from build123d import *

# Parameters (mm, degrees)
BOSS_EXTRUDE1_DEPTH = 3.175
SKETCH4_W           = 17.018
SKETCH4_H           = 3.175
SKETCH4_H_2         = 3.144138513
SKETCH4_W_2         = 3.937
SKETCH4_W_3         = 12.7
CUT_EXTRUDE1_DEPTH  = 3.175
SKETCH5_W           = 7.516860114
SKETCH5_H           = 3.175
CUT_EXTRUDE2_DEPTH  = 3.175
SKETCH6_R           = 1.0287
CUT_EXTRUDE3_DEPTH  = 3.175
CUT_EXTRUDE4_DEPTH  = 4.064


with BuildPart() as part:
    # Sketch2 → Boss-Extrude1 (new body)
    with BuildSketch(Plane.XY):
        Polygon((-71.3232, 6.731), (11.7348, 6.731), (11.7348, 25.781), align=None)
        Polygon((11.7348, 25.781), (11.7348, 6.731), (71.3232, 6.731), align=None)
        Polygon((11.7348, 6.731), (11.7348, -6.731), (71.3232, -6.731), (71.3232, -4.699), (67.2592, -4.699), (67.2592, -1.143), (71.3232, -1.143), (71.3232, 0.381), (67.2592, 0.381), (67.2592, 3.937), (71.3232, 3.937), (71.3232, 4.572927428), (71.3232, 6.731), align=None)
        Polygon((-71.3232, -6.731), (11.7348, -6.731), (11.7348, 6.731), (-71.3232, 6.731), (-71.3232, 3.937), (-67.2592, 3.937), (-67.2592, 0.381), (-71.3232, 0.381), (-71.3232, -1.143), (-67.2592, -1.143), (-67.2592, -4.699), (-71.3232, -4.699), align=None)
    extrude(amount=BOSS_EXTRUDE1_DEPTH)

    # Sketch4 → Cut-Extrude1 (cut)
    with BuildSketch(Plane.XY.offset(3.175)):
        with Locations((-45.7962, -5.1435)):
            Rectangle(SKETCH4_W, SKETCH4_H)
        with Locations((-11.7602, -5.1435)):
            Rectangle(SKETCH4_W, SKETCH4_H)
        with Locations((22.2758, -5.158930744)):
            Rectangle(SKETCH4_W, SKETCH4_H_2)
        with Locations((75.1713, -5.1435)):
            Rectangle(SKETCH4_W_2, SKETCH4_H)
        with Locations((54.1528, -5.158930744)):
            Rectangle(SKETCH4_W_3, SKETCH4_H_2)
    extrude(amount=-CUT_EXTRUDE1_DEPTH, mode=Mode.SUBTRACT)

    # Sketch5 → Cut-Extrude2 (cut)
    with BuildSketch(Plane.XY.offset(3.175)):
        with Locations((68.198230057, -5.1435)):
            Rectangle(SKETCH5_W, SKETCH5_H)
    extrude(amount=-CUT_EXTRUDE2_DEPTH, mode=Mode.SUBTRACT)

    # Sketch6 → Cut-Extrude3 (cut)
    with BuildSketch(Plane.XY.offset(3.175)):
        with Locations((-61.9252, -1.8542)):
            Circle(SKETCH6_R)
        with Locations((-58.378607788, -1.8542)):
            Circle(SKETCH6_R)
        with Locations(Location((61.9252, -1.8542, 0), (0, 0, 180))):
            Circle(SKETCH6_R)
        with Locations(Location((58.378607788, -1.8542, 0), (0, 0, 180))):
            Circle(SKETCH6_R)
    extrude(amount=-CUT_EXTRUDE3_DEPTH, mode=Mode.SUBTRACT)

    # Sketch7 → Cut-Extrude4 (cut)
    with BuildSketch(Plane.XY.offset(3.175)):
        Polygon((-63.896048939, 8.434475014), (-57.706756389, 9.854037525), (-56.996975133, 6.75939125), (-63.186267684, 5.339828739), align=None)
        Polygon((-47.803888308, 12.125337544), (-32.949586187, 15.532287572), (-32.239804931, 12.437641297), (-47.094107052, 9.030691269), align=None)
        Polygon((-23.046718106, 17.80358759), (-16.857425556, 19.223150102), (-16.1476443, 16.128503827), (-22.33693685, 14.708941315), align=None)
        Polygon((-6.954557475, 21.49445012), (-0.765264924, 22.914012632), (-0.055483668, 19.819366357), (-6.244776219, 18.399803845), align=None)
        Polygon((24.145430883, 21.813407007), (30.193862821, 19.879765083), (29.227041859, 16.855549114), (23.178609921, 18.789191038), align=None)
        Polygon((36.242294759, 17.946123159), (42.290726697, 16.012481235), (41.323905735, 12.988265266), (35.275473797, 14.92190719), align=None)
        Polygon((47.129472248, 14.465567696), (53.177904186, 12.531925772), (52.211083224, 9.507709803), (46.162651286, 11.441351727), align=None)
        Polygon((58.016649736, 10.985012233), (64.065081674, 9.051370309), (63.098260712, 6.02715434), (57.049828774, 7.960796264), align=None)
    extrude(amount=-CUT_EXTRUDE4_DEPTH, mode=Mode.SUBTRACT)


solid = part.part
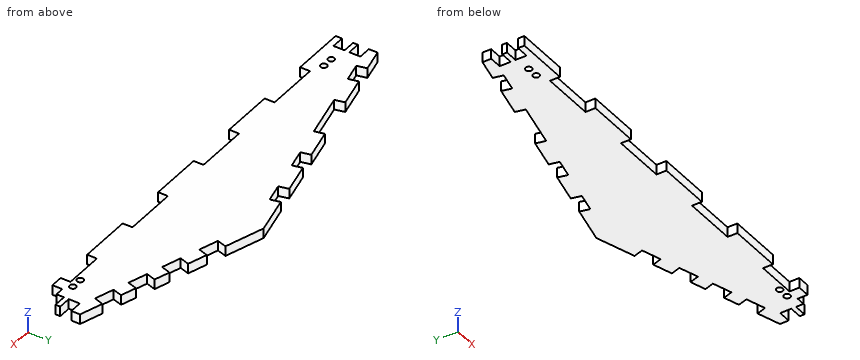
Work out the finished part from the listing and answer in its coordinate system (mm). Give positions to 0.01 mm unless a question says otherwise; leave off trailing zeros. Order: outer loops, then holes, each group sorted by start corner. A loop starts at its lowest first (then second) coordinate and runs counter-clockwise, first axis right, second up. Notation, with made-up numbers: (44, 75) -> (89, 75) arc R11 cw to (89, 80) -> close; hole circle Ø8 at (34.25, 69.5). An arc over 180 degrees is marked (long way). Answer as a JSON object with one key per item and string values. Group by question number.
1. Section A-A on z = 0.65 is taken. Count the separate pieces of the cut face and the enclosed holes in it, plus the area to 3 significant figures.
2. Section B-B on x = 32 is taken. Determine the outline of the cut face in (y, z) (3 decimals).
3. Flat-ended cylindrical pins translate along their axes: pin 1 Ø1.4 at (x, z) = (65.5, 2.5) entering from -Y; pin 2 Ø1.6 at (y, z) = (2.5, 2) entering from +X; pin 3 Ø1 at (y, z) = (1.5, 2) entering from -X. Find the tip coordinate at first contact, or state that the pin passes through.
4. Section C-C on x = -24.5 is taken. Determine the outline of the cut face in (y, z) (3 decimals).
5. Consider line 1 along Y through (x, z) = (-38.5, 0.15); line 2 along X through (y, z) = (0.5, 1.3); line 3 along Y through (x, z) = (0.5, 0.5). Determine where each line is inside the solid, lowest interval first. Write a range as [from, to].
Result sheet:
{
 "1": {"separate pieces": "1", "enclosed holes": "4", "area": "2,800 mm^2"},
 "2": {"outline": "(-6.731, 0) -> (19.302, 0) -> (19.302, 3.175) -> (-6.731, 3.175) -> close"},
 "3": {"pin 1": "stops at y = -3.56", "pin 2": "stops at x = 67.26", "pin 3": "stops at x = -67.26"},
 "4": {"outline": "(-6.731, 0) -> (17.47, 0) -> (17.47, 3.175) -> (-6.731, 3.175) -> close"},
 "5": {"line 1": "y = [-3.56, 11]", "line 2": "x = [-67.26, 67.26]", "line 3": "y = [-6.73, 23.2]"}
}
